The listing builds one solid part. Answer for the finished solid, in the listing's coordinates (mm). A direction names the side the tool comes from. Give positions to 0.01 mm unless a question says otherwise; leave off trailing zeros. Loops run counter-clockwise (first coordinate to the right, second up) from the corner with the lowest first, then second, coordinate; pieces in that order, holes last. Notation, with made-up numbers: (74.25, 10) - (132.25, 10) arc R27 cw to (132.25, 47) - close; hole circle Ø7 at (74, -31). An arc over 180 degrees is marked (long way). Write item = value, one per line. Start each with the question number.
1) The mould has two halves that part along Y. Classify faces 5 (the flat face through (0, 0, 0)), 6 (the flat face through (0, 17, -15)), 7 (the flat face through (9, 76, 9)): +Y half, -Y half, draft (parallel to the pull), parting line (faces both ways), or undercut.
2) Which of the six approach directions +Z, -Z, +X, -X, +Y, -Y give full straight-line access (tool end or side, diameter ignored) to faces 1 (the flat face through (-18.5, 17, 0)), 2 (the cylindrical face through (-2.38, 71.44, 10.74)), 3 (the flat face through (18.5, 17, 0)), 4 (the flat face through (0, 17, 15))?
3) The part is cut by section C-C on z = -23.5. Write down the section's boundary in (x, y), plus the area to 3 significant figures.
4) Flat-ended cylindrical pins translate along their axes: P1, Ø4, axis at y = 31.5, z = -4, coming from the +X side; P2, Ø5, axis at x = -4.5, z = 21.5, coming from the +Y side; P3, Ø8, axis at x = 19.5, y = 53.5, coming from the +Z side; P4, Ø1, axis at x = 3.5, y = 44, coming from the +Z side. Find the tip coordinate at first contact, or state that the pin passes through.
5) Consider probe 1 along Y at (x, z) = (14, 7); probe 2 along Z at (x, y) = (12.5, 10); probe 3 along Y at (x, z) = (-10, 17.5). Determine where each line is inside the solid, lowest interval first.
6) The part is cut by section B-B on y = 26.5. Write down the section's boundary in (x, z).
7) The part is cut by section A-A on x = 16. Write down the section's boundary in (y, z).
from build123d import *

# Parameters (mm, degrees)
ESBO_O1_W                = 37
ESBO_O1_H                = 30
RESSALTO_EXTRUS_O1_DEPTH = 34
ESBO_O2_R                = 11.75
RESSALTO_EXTRUS_O2_DEPTH = 4
ESBO_O3_R                = 14.5
RESSALTO_EXTRUS_O3_DEPTH = 8
ESBO_O4_R                = 13
RESSALTO_EXTRUS_O4_DEPTH = 1
ESBO_O5_R                = 11
RESSALTO_EXTRUS_O5_DEPTH = 5
ESBO_O6_R                = 30
RESSALTO_EXTRUS_O6_DEPTH = 2
ESBO_O7_R                = 14
RESSALTO_EXTRUS_O7_DEPTH = 13
ESBO_O8_R                = 11
RESSALTO_EXTRUS_O8_DEPTH = 9
ESBO_O9_R                = 20
RESSALTO_EXTRUS_O9_DEPTH = 2


with BuildPart() as part:
    # Esboço1 → Ressalto-extrusão1 (new body)
    with BuildSketch(Plane(origin=(0, 0, 0), x_dir=(1, 0, 0), z_dir=(0, 1, 0))):
        Rectangle(ESBO_O1_W, ESBO_O1_H)
    extrude(amount=RESSALTO_EXTRUS_O1_DEPTH)

    # Esboço2 → Ressalto-extrusão2 (add)
    with BuildSketch(Plane(origin=(0, 34, 0), x_dir=(1, 0, 0), z_dir=(0, 1, 0))):
        Circle(ESBO_O2_R)
    extrude(amount=RESSALTO_EXTRUS_O2_DEPTH)

    # Esboço3 → Ressalto-extrusão3 (add)
    with BuildSketch(Plane(origin=(0, 38, 0), x_dir=(1, 0, 0), z_dir=(0, 1, 0))):
        Circle(ESBO_O3_R)
    extrude(amount=RESSALTO_EXTRUS_O3_DEPTH)

    # Esboço4 → Ressalto-extrusão4 (add)
    with BuildSketch(Plane(origin=(0, 46, 0), x_dir=(1, 0, 0), z_dir=(0, 1, 0))):
        Circle(ESBO_O4_R)
    extrude(amount=RESSALTO_EXTRUS_O4_DEPTH)

    # Esboço5 → Ressalto-extrusão5 (add)
    with BuildSketch(Plane(origin=(0, 47, 0), x_dir=(1, 0, 0), z_dir=(0, 1, 0))):
        Circle(ESBO_O5_R)
    extrude(amount=RESSALTO_EXTRUS_O5_DEPTH)

    # Esboço6 → Ressalto-extrusão6 (add)
    with BuildSketch(Plane(origin=(0, 52, 0), x_dir=(1, 0, 0), z_dir=(0, 1, 0))):
        Circle(ESBO_O6_R)
    extrude(amount=RESSALTO_EXTRUS_O6_DEPTH)

    # Esboço7 → Ressalto-extrusão7 (add)
    with BuildSketch(Plane(origin=(0, 54, 0), x_dir=(1, 0, 0), z_dir=(0, 1, 0))):
        Circle(ESBO_O7_R)
    extrude(amount=RESSALTO_EXTRUS_O7_DEPTH)

    # Esboço8 → Ressalto-extrusão8 (add)
    with BuildSketch(Plane(origin=(0, 67, 0), x_dir=(1, 0, 0), z_dir=(0, 1, 0))):
        Circle(ESBO_O8_R)
    extrude(amount=RESSALTO_EXTRUS_O8_DEPTH)

    # Esboço9 → Ressalto-extrusão9 (add)
    with BuildSketch(Plane(origin=(0, 76, 0), x_dir=(1, 0, 0), z_dir=(0, 1, 0))):
        Circle(ESBO_O9_R)
    extrude(amount=RESSALTO_EXTRUS_O9_DEPTH)


solid = part.part
Answer below:
q1.face_5 = -Y half
q1.face_6 = draft
q1.face_7 = undercut
q2.face_1 = +Z, -Z, -X, -Y
q2.face_2 = none
q2.face_3 = +Z, -Z, +X, -Y
q2.face_4 = +Z, +X, -X, -Y
q3.outline = (-18.65, 52) - (18.65, 52) - (18.65, 54) - (-18.65, 54) - close
q3.area = 74.6 mm2
q4.P1 = 18.5
q4.P2 = 78
q4.P3 = 25.69
q4.P4 = 14.19
q5.probe_1 = 0 to 34, 52 to 54, 76 to 78
q5.probe_2 = -15 to 15
q5.probe_3 = 52 to 54
q6.outline = (-18.5, -15) - (18.5, -15) - (18.5, 15) - (-18.5, 15) - close
q7.outline = (0, -15) - (34, -15) - (34, 15) - (0, 15) - close; (52, -25.38) - (54, -25.38) - (54, 25.38) - (52, 25.38) - close; (76, -12) - (78, -12) - (78, 12) - (76, 12) - close
